Autodesk Inventor part; units mm, degrees
ref_plane "Arbeitsebene1" through (0, 0, 160) normal (0, 0, 1) x (1, 0, 0)
ref_plane "YZ Plane" through (0, 0, 0) normal (1, 0, 0) x (0, 1, 0)
ref_plane "XZ Plane" through (0, 0, 0) normal (0, 1, 0) x (-1, 0, 0)
ref_plane "Arbeitsebene1" through (0, 0, 160) normal (0, 0, 1) x (1, 0, 0)
sketch "Skizze2" plane through (0, 0, 160) normal (0, 0, 1) x (1, 0, 0)
  circle A0 centre (0, 0) radius 6
  dimension "d3" = 12
extrude "Extrusion2" add sketch "Skizze2" along normal blind 5
sketch "Skizze3" plane through (0, 0, 160) normal (0, 0, -1) x (-1, 0, 0)
  circle A0 centre (0, 0) radius 3
  dimension "d6" = 6
extrude "Extrusion3" add sketch "Skizze3" along normal blind 170
sketch "Skizze4" plane through (0, 0, 0) normal (0, 1, 0) x (-1, 0, 0)
  line L0 (-3, -10) -> (3, -10)
  line L1 (0, -10) -> (0, 4)
  circle A0 centre (0, -6) radius 1.6
  point P0 (0, 0)
  dimension "d9" = 14
  dimension "d10" = 3.2
extrude "Extrusion4" cut sketch "Skizze4" along normal mid plane 6
properties part number "Bolzen fuer Ruder"
Design review of the part built by this model. Coordinates are the model's own, in mm. A direction names the side the tool comes from. Give positions to 0.01 mm unless a question says otherwise; leave off trailing zeros. Loops run counter-clockwise (first coordinate to the right, second up) from the corner with the lowest first, then second, coordinate; pieces in that order, holes last. Notation, with made-up numbers: M 26,51 L 34,51 A13 ccw 34,56 Z; hole C -32.75,40.5 d11. An arc over 180 degrees is marked long. Return JSON: item names as keys, results as strings. Group by question number.
Item 1: Tool access review of faces 1 (the cylindrical face through (-6, 0, 162)), 2 (the flat face through (-3, -1, 160)): name each direction out of +Z, -Z, +X, -X, +Y, -Y from which nothing blocks a thin tool from reaching the whole face with its end or side.
Item 2: We need section D-D (z = -6). Give the boundary of the cut face in (x, y), and give its area (3 significant figures).
Item 3: Mouldability with a two-part tool opening along X and no side actions: class faces 3 (the cylindrical face through (1.6, 0.04, -5.93)), 4 (the cylindrical face through (3, 0, 76)), 5 (the flat face through (0, 0, 165)) as released by +X, released by -X, zero draft, split by the parting line, or undercut.
Item 4: We need section C-C (z = 19.5). Give the boundary of the cut face in (x, y).
Item 5: Insertion check: pin 1 Ø5 at (x, z) = (0, -6) entering from +Y; pin 2 Ø1.5 at (x, y) = (-2, 4) entering from -Z. Each pin has a flat end and moves straight along its axis. Give the tip position at first contact, or say it passes through.
Item 6: For probe 1 along Z at (x, y) = (3, -4.75); probe 2 along Z at (x, y) = (0, 0); probe 3 along Z at (x, y) = (-1.25, -1), list the stretches that pass through material, from the lowest coordinate up.
Item 7: We need section A-A (x = 0). Give the boundary of the cut face in (y, z).
Item 8: We need section B-B (y = 0). Give the boundary of the cut face in (x, z), and give its area (3 significant figures).
Output:
{
 "1": {"face 1": "+Z, -Z", "face 2": "-Z"},
 "2": {"outline": "M -1.6,-2.54 L -1.6,2.54 A3 ccw Z; M 1.6,-2.54 A3 ccw 1.6,2.54 Z", "area": "10.0 mm^2"},
 "3": {"face 3": "undercut", "face 4": "split by the parting line", "face 5": "zero draft"},
 "4": {"outline": "C 0,0 d6"},
 "5": {"pin 1": "stops at y = 3", "pin 2": "stops at z = 160"},
 "6": {"probe 1": "z = 160 to 165", "probe 2": "z = -10 to -7.6, -4.4 to 165", "probe 3": "z = -10 to -7, -5 to 165"},
 "7": {"outline": "M -6,160 L -3,160 L -3,-4.4 L 3,-4.4 L 3,160 L 6,160 L 6,165 L -6,165 Z; M -3,-10 L 3,-10 L 3,-7.6 L -3,-7.6 Z"},
 "8": {"outline": "M -6,160 L -3,160 L -3,-10 L 3,-10 L 3,160 L 6,160 L 6,165 L -6,165 Z; hole C 0,-6 d3.2", "area": "1,070 mm^2"}
}
